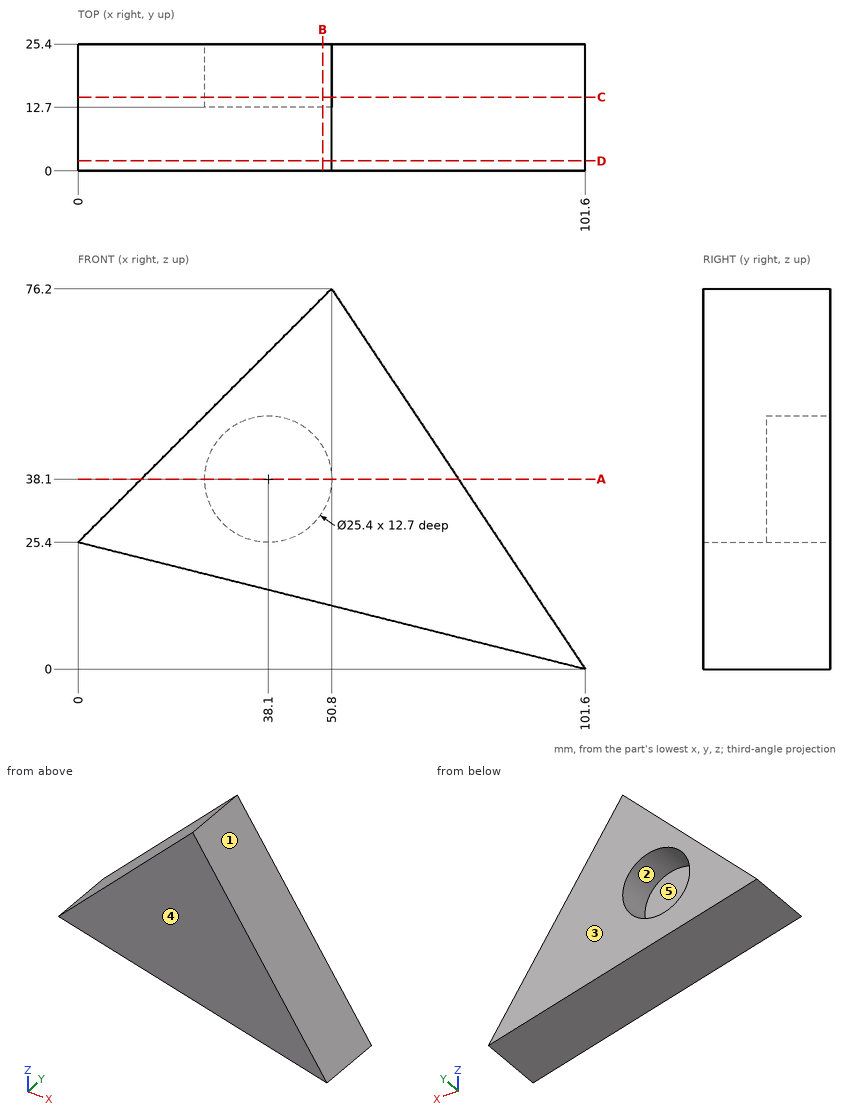
Study the drawing (mm; zero at the part's minimum x, y, z) and answer. A direction names the side the tool comes from. Give positions to 0.01 mm unless a question says otherwise; leave off trailing zeros. Loops run counter-clockwise (first coordinate to the right, second up) from the corner with the lowest first, then second, coordinate; pieces in that order, holes last. Notation, with made-up numbers: M -11,33 L 22,33 A21 ccw 22,65 Z; hole C 37,46 d8. An arc over 180 degrees is marked long. One line per item, written item: value.
1. For the marked faces 4 and 5, determine the directions among +Z, -Z, +X, -X, +Y, -Y from which every point of the face is accessible in a straight line to the end or side of a thin tool.
Found:
face 4: +Z, -Z, +X, -X, -Y
face 5: +Y
2. Find the intervals of material crossed by probe 1 along Z at (x, y) = (38.1, 21.75) (3 decimals); probe 2 along Z at (x, y) = (35.5, 15.5) (3 decimals); probe 3 along Z at (x, y) = (41.5, 2.5) (3 decimals), in increasing order.
Found:
probe 1: 15.875 to 25.4, 50.8 to 63.5
probe 2: 16.525 to 25.669, 50.531 to 60.9
probe 3: 15.025 to 66.9
3. For a pull along X with two mould halves and no side action, classify the marked faces 1, 2 and 3 as pulls with the +X half, pulls with the -X half, needs draft (parallel to the pull), parting line crosses it, or undercut.
Found:
face 1: pulls with the +X half
face 2: undercut
face 3: needs draft
4. Section D-D on y = 2 is taken. Determine the outline of the cut face in (x, z).
Found:
outline: M 0,25.4 L 101.6,0 L 50.8,76.2 Z
5. Section C-C on y = 14.75 is taken. Determine the outline of the cut face in (x, z), plus the area to 3 significant figures.
Found:
outline: M 0,25.4 L 101.6,0 L 50.8,76.2 Z; hole C 38.1,38.1 d25.4
area: 2,720 mm^2
6. Section B-B on x = 49 is taken. Determine the outline of the cut face in (y, z), plus the area to 3 significant figures.
Found:
outline: M 0,13.15 L 25.4,13.15 L 25.4,31.58 L 12.7,31.58 L 12.7,44.62 L 25.4,44.62 L 25.4,74.4 L 0,74.4 Z
area: 1,390 mm^2
7. Each of these flat-tipped pins is pushed along its axis until it touches: P1, Ø4, axis at y = 11, z = 22.5, coming from the +X side; P2, Ø7.5, axis at x = 39, z = 42.5, coming from the +Y side; P3, Ø5, axis at y = 8.5, z = 58.5, coming from the -X side. Where does it stop, or does it pass through?
Found:
P1: x = 87.93
P2: y = 12.7
P3: x = 30.6
8. Section A-A on z = 38.1 is taken. Determine the outline of the cut face in (x, y).
Found:
outline: M 12.7,0 L 76.2,0 L 76.2,25.4 L 50.8,25.4 L 50.8,12.7 L 25.4,12.7 L 25.4,25.4 L 12.7,25.4 Z
